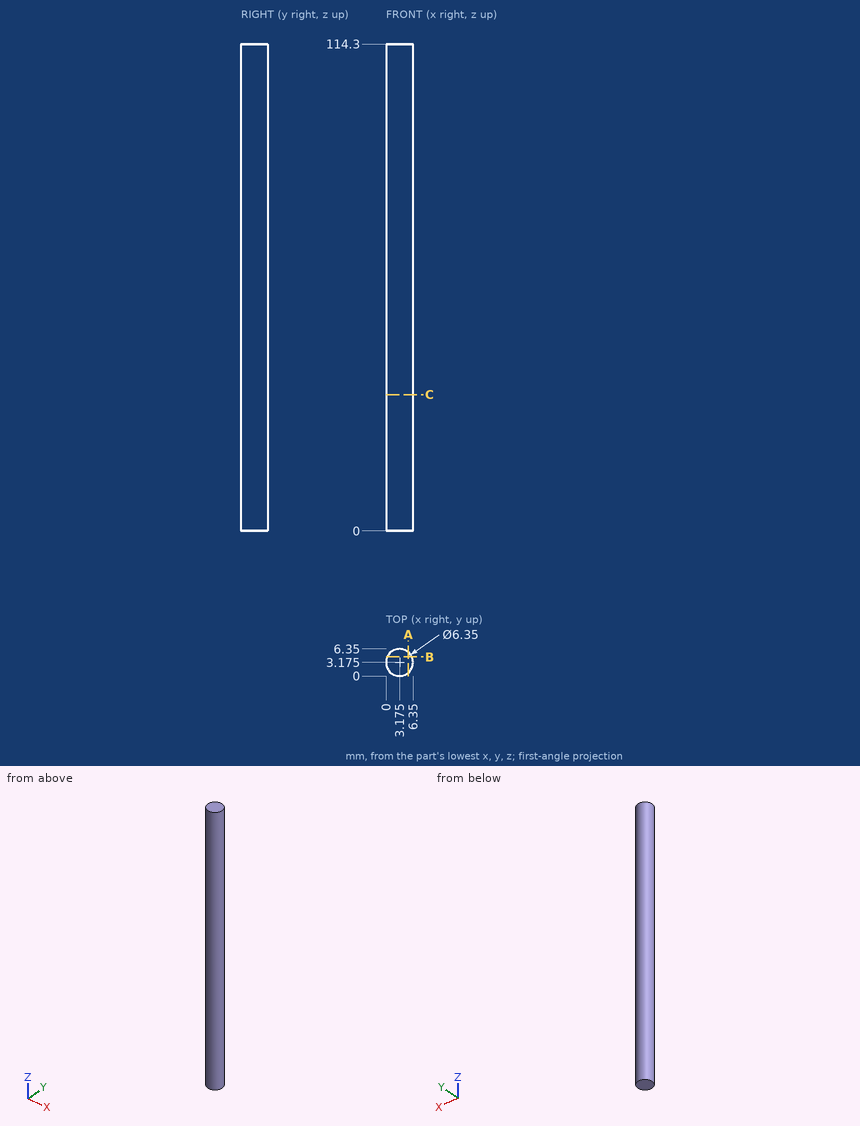
Could you check a few things on this drawing? It's one solid part, dimensions in mm from its lowest x, y, z. Round coordinates to 2 decimals unless told otherwise and drop trailing zeros. Loops run counter-clockwise (first coordinate to the right, second up) from the corner with the lowest first, then second, coordinate; pieces in that order, holes last. Notation, with made-up numbers: (62.25, 82.5) -> (68.25, 82.5) arc R35 cw to (68.25, 116.5) -> close; hole circle Ø2 at (66.25, 51.25). An arc over 180 degrees is marked (long way). One line per item, written item: value. Start each with the question number.
1. If we section it at A-A, the plane x = 5.25: Write out the boundary of the cut face in (y, z), then the cut area to 3 significant figures.
2. If we section it at B-B, the plane y = 4.5: Write out the boundary of the cut face in (x, z).
3. If I drill on probe 1 along X at (y, z) = (3.5, 38.5); probe 2 along X at (y, z) = (5.5, 54.5); probe 3 along Y at (x, z) = (2.25, 52), over which ranges is the centre line in solid material (lowest first)?
4. If we section it at C-C, the plane z = 32: Write out the boundary of the cut face in (x, y) (3 decimals).
Calculated:
1. outline: (0.77, 0) -> (5.58, 0) -> (5.58, 114.3) -> (0.77, 114.3) -> close
1. area: 549 mm²
2. outline: (0.29, 0) -> (6.06, 0) -> (6.06, 114.3) -> (0.29, 114.3) -> close
3. probe 1: x = 0.02 to 6.33
3. probe 2: x = 1.01 to 5.34
3. probe 3: y = 0.14 to 6.21
4. outline: circle Ø6.35 at (3.175, 3.175)
